Here's how the part is built. I have some questions about the finished solid (model axes, mm). Face numbers are marked on the shaded views. A direction names the side the tool comes from. Round coordinates to 2 decimals unless told otherwise and drop trailing zeros. Write each loop counter-clockwise with the first axis right and the second up, starting at its lowest first coordinate (ties: lowest second). Pieces come first, ordered by that corner, then holes. Notation, with made-up numbers: M 50,61 L 72,61 A11 cw 72,77 Z; hole C 18,-9.5 d5. An arc over 180 degrees is marked long. Use one line per item in the form item = value. Start each with the question number.
Q1. For the marked faces 1, 2 and 3, which set-ups out of +Z, -Z, +X, -X, +Y, -Y let a thin tool reach every point of the face, with its end or its side?
Q2. I want a section at C-C on y = -6.5. List the corners of the cut face in (x, z) for me.
Q3. I want a section at D-D on z = 44. List the corners of the cut face in (x, y) for me, and give its area (3 significant figures).
Q4. I want a section at B-B on y = 19.05. List the corners of the cut face in (x, z) for me, and give its area (3 significant figures).
Q5. I want a section at A-A on x = -209.55. List the corners of the cut face in (y, z) for me, and give its area (3 significant figures).
Q6. I'm going to push flat-ended pins straight in: pin 1 Ø11 at (x, y) = (-209.55, -19.05) entering from -Z; pin 2 Ø19 at (x, y) = (198.5, -4) entering from +Z; pin 3 Ø9.5 at (y, z) = (18.5, 49.5) entering from -X. Where does each tip first touch, or does it pass through?
Q7. I need wall thicknesses on line 1 along Y through (x, z) = (209, 15); line 2 along X through (y, z) = (19, 13); line 3 along X through (y, z) = (8.5, 50.5). Which ranges of each line are inside material? Lowest first, please. Write a range as from..to.
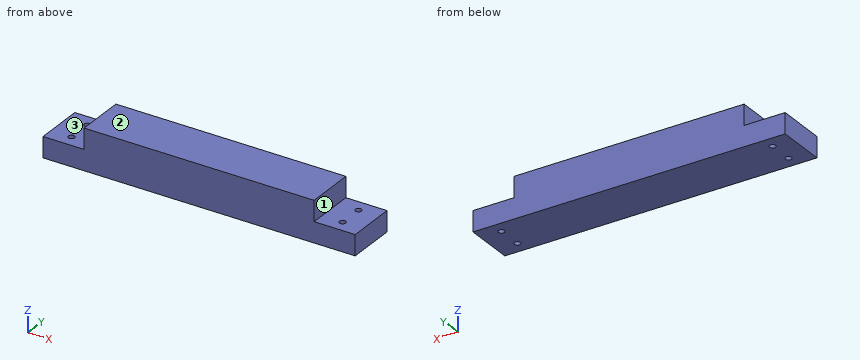
```python
from build123d import *

# Parameters (mm, degrees)
SKETCH1_W           = 482.6
SKETCH1_H           = 76.2
BOSS_EXTRUDE1_DEPTH = 31.75
SKETCH2_W           = 355.6
SKETCH2_H           = 76.2
BOSS_EXTRUDE2_DEPTH = 31.75
SKETCH3_R           = 4.7625
CUT_EXTRUDE1_DEPTH  = 247.343992214


with BuildPart() as part:
    # Sketch1 → Boss-Extrude1 (new body)
    with BuildSketch(Plane.XY):
        Rectangle(SKETCH1_W, SKETCH1_H)
    extrude(amount=BOSS_EXTRUDE1_DEPTH)

    # Sketch2 → Boss-Extrude2 (add)
    with BuildSketch(Plane.XY.offset(31.75)):
        Rectangle(SKETCH2_W, SKETCH2_H)
    extrude(amount=BOSS_EXTRUDE2_DEPTH)

    # Sketch3 → Cut-Extrude1 (cut, through all)
    with BuildSketch(Plane.XY.offset(31.75)):
        with Locations((-209.55, 19.05)):
            Circle(SKETCH3_R)
        with Locations((-209.55, -19.05)):
            Circle(SKETCH3_R)
    cut_extrude1 = extrude(amount=-CUT_EXTRUDE1_DEPTH, mode=Mode.SUBTRACT)

    # Mirror1: Cut-Extrude1 across plane
    add(cut_extrude1.mirror(Plane(origin=(0, 0, 0), x_dir=(0, 0, 1), z_dir=(1, 0, 0))), mode=Mode.SUBTRACT)


solid = part.part
```
Reported:
q1.face_1 = +Z, +X, +Y, -Y
q1.face_2 = +Z, +X, -X, +Y, -Y
q1.face_3 = +Z, -X, +Y, -Y
q2.outline = M -241.3,0 L 241.3,0 L 241.3,31.75 L 177.8,31.75 L 177.8,63.5 L -177.8,63.5 L -177.8,31.75 L -241.3,31.75 Z
q3.outline = M -177.8,-38.1 L 177.8,-38.1 L 177.8,38.1 L -177.8,38.1 Z
q3.area = 27,100 mm^2
q4.outline = M -241.3,0 L -214.31,0 L -214.31,31.75 L -241.3,31.75 Z; M -204.79,0 L 204.79,0 L 204.79,31.75 L 177.8,31.75 L 177.8,63.5 L -177.8,63.5 L -177.8,31.75 L -204.79,31.75 Z; M 214.31,0 L 241.3,0 L 241.3,31.75 L 214.31,31.75 Z
q4.area = 26,000 mm^2
q5.outline = M -38.1,0 L -23.81,0 L -23.81,31.75 L -38.1,31.75 Z; M -14.29,0 L 14.29,0 L 14.29,31.75 L -14.29,31.75 Z; M 23.81,0 L 38.1,0 L 38.1,31.75 L 23.81,31.75 Z
q5.area = 1,810 mm^2
q6.pin_1 = 0
q6.pin_2 = 31.75
q6.pin_3 = -177.8
q7.line_1 = -38.1..-23.78, -14.32..14.32, 23.78..38.1
q7.line_2 = -241.3..-214.31, -204.79..204.79, 214.31..241.3
q7.line_3 = -177.8..177.8
